Source: CAD feature listing. Evaluate the final solid. Frame: model axes, mm. Give positions to 0.01 mm unless a question says otherwise; leave off trailing zeros. Order: outer loops, then holes, each group sorted by start corner. A loop starts at its lowest first (then second) coordinate and runs counter-clockwise, first axis right, second up. Notation, with made-up numbers: (-30, 57.5) -> (-14, 57.5) arc R17 cw to (-14, 89.5) -> close; hole circle Ø9 at (24.25, 52). An arc over 180 degrees is marked (long way). Answer in a Markdown table with one row per item.
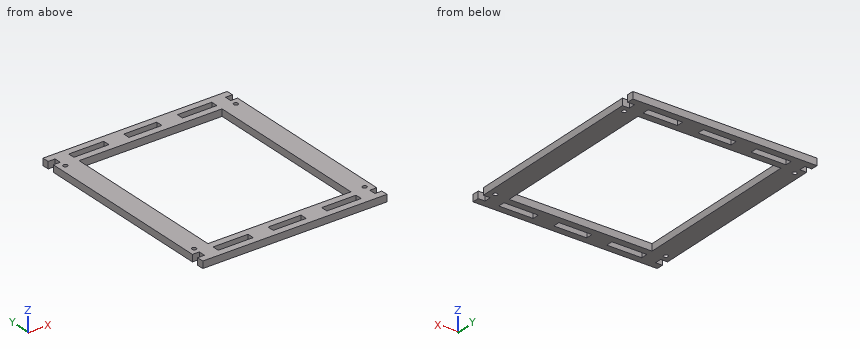
Autodesk Inventor part; units mm, degrees
ref_plane "YZ Plane" through (0, 0, 0) normal (1, 0, 0) x (0, 1, 0)
ref_plane "XZ Plane" through (0, 0, 0) normal (0, 1, 0) x (-1, 0, 0)
ref_plane "XY Plane" through (0, 0, 0) normal (0, 0, 1) x (1, 0, 0)
sketch "Sketch1" plane through (0, 0, 0) normal (0, 0, 1) x (1, 0, 0)
  line L0 (-22.2313, 26.7915) -> (109.8487, 26.7915)
  line L1 (109.8487, 26.7915) -> (109.8487, -144.6585)
  line L2 (109.8487, -144.6585) -> (-22.2313, -144.6585)
  line L3 (-22.2313, -144.6585) -> (-22.2313, 26.7915)
  line L4 (-22.2313, 26.7915) -> (-28.5813, 26.7915)
  line L5 (-28.5813, 26.7915) -> (-28.5813, 39.4915)
  line L6 (-28.5813, 39.4915) -> (116.1987, 39.4915)
  line L7 (116.1987, 39.4915) -> (116.1987, 26.7915)
  line L8 (116.1987, 26.7915) -> (128.8987, 26.7915)
  line L9 (128.8987, 26.7915) -> (128.8987, 14.0915)
  line L10 (128.8987, 14.0915) -> (116.1987, 14.0915)
  line L11 (116.1987, 14.0915) -> (116.1987, -131.9585)
  line L12 (116.1987, -131.9585) -> (128.8987, -131.9585)
  line L13 (128.8987, -131.9585) -> (128.8987, -144.6585)
  line L14 (128.8987, -144.6585) -> (116.1987, -144.6585)
  line L15 (116.1987, -144.6585) -> (116.1987, -154.1835)
  line L16 (116.1987, -154.1835) -> (-28.5813, -154.1835)
  line L17 (-28.5813, -154.1835) -> (-28.5813, -144.6585)
  line L18 (-28.5813, -144.6585) -> (-41.2813, -144.6585)
  line L19 (-41.2813, -144.6585) -> (-41.2813, -131.9585)
  line L20 (-41.2813, -131.9585) -> (-28.5813, -131.9585)
  line L21 (-28.5813, -131.9585) -> (-28.5813, 14.0915)
  line L22 (-28.5813, 14.0915) -> (-41.2813, 14.0915)
  line L23 (-41.2813, 14.0915) -> (-41.2813, 26.7915)
  line L24 (-41.2813, 26.7915) -> (-28.5813, 26.7915)
  line L25 (-22.2313, -144.6585) -> (-22.2313, -151.0085)
  line L26 (-22.2313, -151.0085) -> (15.8687, -151.0085)
  line L27 (15.8687, -151.0085) -> (15.8687, -144.6585)
  line L28 (15.8687, -144.6585) -> (22.2187, -144.6585)
  line L29 (22.2187, -144.6585) -> (22.2187, -151.0085)
  line L30 (109.8487, -144.6585) -> (109.8487, -151.0085)
  line L31 (109.8487, -151.0085) -> (71.7487, -151.0085)
  line L32 (71.7487, -151.0085) -> (71.7487, -144.6585)
  line L33 (71.7487, -144.6585) -> (65.3987, -144.6585)
  line L34 (65.3987, -144.6585) -> (65.3987, -151.0085)
  line L35 (65.3987, -151.0085) -> (22.2187, -151.0085)
  line L36 (-22.2313, 26.7915) -> (-22.2313, 33.1415)
  line L37 (-22.2313, 33.1415) -> (15.8687, 33.1415)
  line L38 (15.8687, 33.1415) -> (15.8687, 26.7915)
  line L39 (22.2187, 26.7915) -> (22.2187, 33.1415)
  line L40 (22.2187, 33.1415) -> (65.3987, 33.1415)
  line L41 (65.3987, 33.1415) -> (65.3987, 26.7915)
  line L42 (71.7487, 26.7915) -> (71.7487, 33.1415)
  line L43 (71.7487, 33.1415) -> (109.8487, 33.1415)
  line L44 (109.8487, 33.1415) -> (109.8487, 26.7915)
  circle A0 centre (-34.9313, 20.4415) radius 1.9812
  circle A1 centre (122.5487, 20.4415) radius 1.9812
  circle A2 centre (122.5487, -138.3085) radius 1.9812
  circle A3 centre (-34.9313, -138.3085) radius 1.9812
  point P0 (0, 0)
  dimension "d0" = 132.08
  dimension "d1" = 171.45
  dimension "d2" = 6.35
  dimension "d3" = 12.7
  dimension "d4" = 144.78
  dimension "d5" = 12.7
  dimension "d6" = 12.7
  dimension "d7" = 146.05
  dimension "d8" = 9.525
  dimension "d9" = 12.7
  dimension "d10" = 6.35
  dimension "d11" = 38.1
  dimension "d12" = 6.35
  dimension "d13" = 38.1
  dimension "d14" = 6.35
  dimension "d15" = 3.9624
  dimension "d16" = 3.9624
extrude "Extrusion1" add sketch "Sketch1" along normal blind 6.35
sketch "Sketch2" plane through (-28.5813, -154.1835, 0) normal (0, -1, 0) x (1, 0, 0)
  line L0 (144.78, 6.35) -> (0, 6.35)
  line L1 (0, 0) -> (0, 6.35)
  line L2 (0, 0) -> (144.78, 0)
  line L3 (144.78, 0) -> (144.78, 6.35)
  point P0 (28.5813, 0)
extrude "Extrusion2" add sketch "Sketch2" along normal blind 3.175
sketch "Sketch3" plane through (0, 0, 6.35) normal (0, 0, 1) x (1, 0, 0)
  line L0 (-28.5813, 14.0915) -> (-41.2813, 14.0915)
  line L1 (-28.5813, -131.9585) -> (-28.5813, 14.0915)
  line L2 (-41.2813, -131.9585) -> (-28.5813, -131.9585)
  line L3 (116.1987, -131.9585) -> (128.8987, -131.9585)
  line L4 (116.1987, 14.0915) -> (116.1987, -131.9585)
  line L5 (128.8987, 14.0915) -> (116.1987, 14.0915)
  line L6 (71.7487, 33.1415) -> (109.8487, 33.1415)
  line L7 (-41.2813, 14.0915) -> (-41.2813, -131.9585)
  line L8 (128.8987, 14.0915) -> (128.8987, -131.9585)
  point P0 (0, 0)
extrude "Extrusion3" add sketch "Sketch3" against normal blind 6.35
sketch "Sketch4" plane through (0, 0, 6.35) normal (0, 0, 1) x (1, 0, 0)
  line L0 (-28.5813, -157.3585) -> (-28.5813, -144.6585)
  line L1 (-28.5813, -157.3585) -> (116.1987, -157.3585)
  line L2 (116.1987, -144.6585) -> (116.1987, -157.3585)
  line L3 (109.8487, 33.1415) -> (109.8487, -151.0085)
  line L4 (-22.2313, -151.0085) -> (-22.2313, 33.1415)
  line L5 (15.8687, 26.7915) -> (22.2187, 26.7915)
  line L6 (71.7487, 33.1415) -> (109.8487, 33.1415)
  line L7 (15.8687, 26.7915) -> (-22.2313, 26.7915)
  line L8 (22.2187, 26.7915) -> (109.8487, 26.7915)
  line L9 (109.8487, 26.7915) -> (109.8487, 20.4415)
  line L10 (109.8487, 20.4415) -> (-22.2313, 20.4415)
  line L11 (-22.2313, 20.4415) -> (-22.2313, 26.7915)
  line L12 (-22.2313, -144.6585) -> (-22.2313, -138.3085)
  line L13 (-22.2313, -138.3085) -> (109.8487, -138.3085)
  line L14 (109.8487, -144.6585) -> (-22.2313, -144.6585)
  line L15 (-28.5813, -151.0085) -> (-41.2813, -151.0085)
  line L16 (-41.2813, -151.0085) -> (-41.2813, -157.3585)
  line L17 (-41.2813, -157.3585) -> (-28.5813, -157.3585)
  line L18 (116.1987, -151.0085) -> (128.8987, -151.0085)
  line L19 (128.8987, -151.0085) -> (128.8987, -157.3585)
  line L20 (128.8987, -157.3585) -> (116.1987, -157.3585)
  point P0 (0, 0)
extrude "Extrusion4" add sketch "Sketch4" against normal blind 6.35 contours L17 L16 L15 L0 | L2 L18 L19 L20 | L3 L10 L4 L7 L5 L8 | L3 L14 L4 L13
sketch "Sketch5" plane through (0, 0, 6.35) normal (0, 0, 1) x (1, 0, 0)
  line L0 (-28.5813, 26.7915) -> (-28.5813, 39.4915)
  line L1 (116.1987, 39.4915) -> (116.1987, 26.7915)
  line L2 (15.8687, 33.1415) -> (15.8687, 26.7915)
  line L3 (-28.5813, 39.4915) -> (-41.2813, 39.4915)
  line L4 (-41.2813, 39.4915) -> (-41.2813, 33.1415)
  line L5 (-41.2813, 33.1415) -> (-28.5813, 33.1415)
  line L6 (116.1987, 39.4915) -> (128.8987, 39.4915)
  line L7 (128.8987, 39.4915) -> (128.8987, 33.1415)
  line L8 (128.8987, 33.1415) -> (116.1987, 33.1415)
  point P0 (0, 0)
extrude "Extrusion5" add sketch "Sketch5" against normal blind 6.35
sketch "Sketch6" plane through (0, 0, 6.35) normal (0, 0, 1) x (1, 0, 0)
  line L0 (65.3987, -151.0085) -> (22.2187, -151.0085)
  line L1 (22.2187, -144.6585) -> (65.3987, -144.6585)
  line L2 (-22.2313, -144.6585) -> (15.8687, -144.6585)
  line L3 (109.8487, -151.0085) -> (71.7487, -151.0085)
  line L4 (65.3987, 26.7915) -> (22.2187, 26.7915)
  line L5 (109.8487, 26.7915) -> (71.7487, 26.7915)
  line L6 (-41.2813, 26.7915) -> (-28.5813, 26.7915)
  line L7 (-28.5813, -151.0085) -> (-41.2813, -151.0085)
  line L8 (128.8987, -151.0085) -> (116.1987, -151.0085)
  line L9 (116.1987, 26.7915) -> (128.8987, 26.7915)
  line L10 (-28.5813, 33.1415) -> (-34.9313, 33.1415)
  line L11 (-34.9313, 33.1415) -> (-34.9313, 26.7915)
  line L12 (-34.9313, 26.7915) -> (-28.5813, 26.7915)
  line L13 (-28.5813, 26.7915) -> (-28.5813, 33.1415)
  line L14 (15.8687, 33.1415) -> (10.0792, 33.1415)
  line L15 (10.0792, 33.1415) -> (10.0792, 26.7915)
  line L16 (10.0792, 26.7915) -> (15.8687, 26.7915)
  line L17 (15.8687, 26.7915) -> (15.8687, 33.1415)
  line L18 (22.2187, 33.1415) -> (28.5687, 33.1415)
  line L19 (28.5687, 33.1415) -> (28.5687, 26.7915)
  line L20 (28.5687, 26.7915) -> (22.2187, 26.7915)
  line L21 (22.2187, 26.7915) -> (22.2187, 33.1415)
  line L22 (65.3987, 33.1415) -> (59.0487, 33.1415)
  line L23 (59.0487, 33.1415) -> (59.0487, 26.7915)
  line L24 (59.0487, 26.7915) -> (65.3987, 26.7915)
  line L25 (65.3987, 26.7915) -> (65.3987, 33.1415)
  line L26 (71.7487, 33.1415) -> (78.0987, 33.1415)
  line L27 (78.0987, 33.1415) -> (78.0987, 26.7915)
  line L28 (78.0987, 26.7915) -> (71.7487, 26.7915)
  line L29 (71.7487, 26.7915) -> (71.7487, 33.1415)
  line L30 (116.1987, 33.1415) -> (122.5487, 33.1415)
  line L31 (122.5487, 33.1415) -> (122.5487, 26.7915)
  line L32 (122.5487, 26.7915) -> (116.1987, 26.7915)
  line L33 (116.1987, 26.7915) -> (116.1987, 33.1415)
  line L34 (-28.5813, -144.6585) -> (-34.9313, -144.6585)
  line L35 (-34.9313, -144.6585) -> (-34.9313, -151.0085)
  line L36 (-34.9313, -151.0085) -> (-28.5813, -151.0085)
  line L37 (-28.5813, -151.0085) -> (-28.5813, -144.6585)
  line L38 (10.0792, -144.6585) -> (28.5687, -144.6585)
  line L39 (28.5687, -144.6585) -> (28.5687, -151.0085)
  line L40 (28.5687, -151.0085) -> (10.0792, -151.0085)
  line L41 (10.0792, -151.0085) -> (10.0792, -144.6585)
  line L42 (59.0487, -144.6585) -> (78.0987, -144.6585)
  line L43 (78.0987, -144.6585) -> (78.0987, -151.0085)
  line L44 (78.0987, -151.0085) -> (59.0487, -151.0085)
  line L45 (59.0487, -151.0085) -> (59.0487, -144.6585)
  line L46 (116.1987, -144.6585) -> (122.5487, -144.6585)
  line L47 (122.5487, -144.6585) -> (122.5487, -151.0085)
  line L48 (122.5487, -151.0085) -> (116.1987, -151.0085)
  line L49 (116.1987, -151.0085) -> (116.1987, -144.6585)
  point P0 (0, 0)
  dimension "d27" = 6.35
  dimension "d28" = 6.35
  dimension "d29" = 6.35
  dimension "d30" = 6.35
  dimension "d31" = 6.35
extrude "Extrusion6" add sketch "Sketch6" against normal blind 6.35 contours L0 L45 L1 L42 L43 L3 L44 | L0 L40 L41 L2 L38 L1 L39 | L4 L21 L18 L19 | L4 L23 L22 L25 | L5 L29 L26 L27 | L11 L10 L13 L6 | L7 L35 L34 L37 | L8 L49 L46 L47 | L33 L30 L31 L9 | L17 L16 L15 L14
properties part number "top-bot connector"
(1) First-contact query: pin 1 Ø1.9 at (y, z) = (30.5, 2) entering from -X. Flat tip, straight axial feed; report the tip coordinate or a pass-through.
A:
| item | result |
|---|---|
| pin 1 | stops at x = -34.93 |
(2) Section query B-B (y = -117). Return the cut outline in (x, z).
A:
| item | result |
|---|---|
| outline | (-41.28, 0) -> (-22.23, 0) -> (-22.23, 6.35) -> (-41.28, 6.35) -> close; (109.85, 0) -> (128.9, 0) -> (128.9, 6.35) -> (109.85, 6.35) -> close |
(3) Ray query, probe 1 along Y at (x, z) = (42, 6.25); probe 2 along X at (y, z) = (-38, 3.5); probe 3 along Y at (x, z) = (24, 3). Return the intervals inside material, ascending.
A:
| item | result |
|---|---|
| probe 1 | y = -157.36 to -151.01, -144.66 to -138.31, 20.44 to 26.79, 33.14 to 39.49 |
| probe 2 | x = -41.28 to -22.23, 109.85 to 128.9 |
| probe 3 | y = -157.36 to -138.31, 20.44 to 39.49 |
(4) Section query A-A (x = 47). Return the cut outline in (y, z).
A:
| item | result |
|---|---|
| outline | (-157.36, 0) -> (-151.01, 0) -> (-151.01, 6.35) -> (-157.36, 6.35) -> close; (-144.66, 0) -> (-138.31, 0) -> (-138.31, 6.35) -> (-144.66, 6.35) -> close; (20.44, 0) -> (26.79, 0) -> (26.79, 6.35) -> (20.44, 6.35) -> close; (33.14, 0) -> (39.49, 0) -> (39.49, 6.35) -> (33.14, 6.35) -> close |
(5) Section query C-C (x = 20). Return the cut outline in (y, z), plus the area to 3 significant figures.
A:
| item | result |
|---|---|
| outline | (-157.36, 0) -> (-138.31, 0) -> (-138.31, 6.35) -> (-157.36, 6.35) -> close; (20.44, 0) -> (39.49, 0) -> (39.49, 6.35) -> (20.44, 6.35) -> close |
| area | 242 mm^2 |
(6) Section query D-D (z = 1.75). Give the number of separate pieces and of enclosed holes in the cut face, plus the area to 3 significant figures.
A:
| item | result |
|---|---|
| separate pieces | 1 |
| enclosed holes | 11 |
| area | 11,100 mm^2 |
